Part model, mm, in its own coordinate system. Coordinates: 2 decimals unless noted, no trailing zeros. Order: outer loops, then holes, each group sorted by start corner. A loop starts at its lowest first (then second) coordinate and runs counter-clockwise, first axis right, second up. Notation, with made-up numbers: M 3,-27 L 29,-27 A30 ccw 29,0 Z; hole C 9,-17.75 d11. An arc over 180 degrees is marked long. Answer in a Markdown table with one row per item. Add a question column.
from build123d import *

# Parameters (mm, degrees)
SKETCH1_W               = 279.4
SKETCH1_H               = 76.2
BOSS_EXTRUDE1_DEPTH     = 3
SKETCH3_W               = 3
SKETCH3_H               = 7.8
CUT_EXTRUDE1_DEPTH      = 145.833352512
LPATTERN1_COUNT         = 4
LPATTERN1_PITCH         = 22.8
MIRROR1_COPY_1_SKETCH_W = 3
MIRROR1_COPY_1_SKETCH_H = 7.8
MIRROR1_COPY_1_DEPTH    = 145.833352512
MIRROR1_COPY_2_SKETCH_W = 3
MIRROR1_COPY_2_SKETCH_H = 7.8
MIRROR1_COPY_2_DEPTH    = 145.833352512
MIRROR1_COPY_3_SKETCH_W = 3
MIRROR1_COPY_3_SKETCH_H = 7.8
MIRROR1_COPY_3_DEPTH    = 145.833352512
SKETCH5_W               = 3
SKETCH5_H               = 15
CUT_EXTRUDE3_DEPTH      = 10
SKETCH9_W               = 3
SKETCH9_H               = 7.8
BOSS_EXTRUDE2_DEPTH     = 3
LPATTERN4_COUNT         = 12
LPATTERN4_PITCH         = 22.8


with BuildPart() as part:
    # Sketch1 → Boss-Extrude1 (new body)
    with BuildSketch(Plane(origin=(0, 0, 0), x_dir=(0, 0, -1), z_dir=(1, 0, 0))):
        Rectangle(SKETCH1_W, SKETCH1_H)
    extrude(amount=-BOSS_EXTRUDE1_DEPTH)

    # Sketch3 → Cut-Extrude1 (cut, through all)
    with BuildSketch(Plane.ZY.offset(3)):
        with Locations((-138.2, 34.2)):
            Rectangle(SKETCH3_W, SKETCH3_H)
    cut_extrude1 = extrude(amount=-CUT_EXTRUDE1_DEPTH, mode=Mode.SUBTRACT)

    # LPattern1: Cut-Extrude1 ×4
    with Locations(*[(0, -i * LPATTERN1_PITCH, 0) for i in range(1, LPATTERN1_COUNT)]):
        add(cut_extrude1, mode=Mode.SUBTRACT)

    # Mirror1: Cut-Extrude1 across plane
    add(cut_extrude1.mirror(Plane.XY), mode=Mode.SUBTRACT)

    # Mirror1 copy 1 sketch → Mirror1 copy 1 (cut, through all)
    with BuildSketch(Plane(origin=(-3, -22.8, 0), x_dir=(0, 0, -1), z_dir=(-1, 0, 0))):
        with Locations((-138.2, -34.2)):
            Rectangle(MIRROR1_COPY_1_SKETCH_W, MIRROR1_COPY_1_SKETCH_H)
    extrude(amount=-MIRROR1_COPY_1_DEPTH, mode=Mode.SUBTRACT)

    # Mirror1 copy 2 sketch → Mirror1 copy 2 (cut, through all)
    with BuildSketch(Plane(origin=(-3, -45.6, 0), x_dir=(0, 0, -1), z_dir=(-1, 0, 0))):
        with Locations((-138.2, -34.2)):
            Rectangle(MIRROR1_COPY_2_SKETCH_W, MIRROR1_COPY_2_SKETCH_H)
    extrude(amount=-MIRROR1_COPY_2_DEPTH, mode=Mode.SUBTRACT)

    # Mirror1 copy 3 sketch → Mirror1 copy 3 (cut, through all)
    with BuildSketch(Plane(origin=(-3, -68.4, 0), x_dir=(0, 0, -1), z_dir=(-1, 0, 0))):
        with Locations((-138.2, -34.2)):
            Rectangle(MIRROR1_COPY_3_SKETCH_W, MIRROR1_COPY_3_SKETCH_H)
    extrude(amount=-MIRROR1_COPY_3_DEPTH, mode=Mode.SUBTRACT)

    # Sketch5 → Cut-Extrude3 (cut)
    with BuildSketch(Plane.ZY.offset(3)):
        with Locations((-21.5, 22.8)):
            Rectangle(SKETCH5_W, SKETCH5_H)
    cut_extrude3 = extrude(amount=-CUT_EXTRUDE3_DEPTH, mode=Mode.SUBTRACT)

    # Mirror2: Cut-Extrude3 across plane
    add(cut_extrude3.mirror(Plane.XY), mode=Mode.SUBTRACT)

    # Sketch9 → Boss-Extrude2 (add)
    with BuildSketch(Plane(origin=(0, 38.1, 0), x_dir=(1, 0, 0), z_dir=(0, 1, 0))):
        with Locations((-1.5, 125.4)):
            Rectangle(SKETCH9_W, SKETCH9_H)
    boss_extrude2 = extrude(amount=BOSS_EXTRUDE2_DEPTH)

    # LPattern4: Boss-Extrude2 ×12
    with Locations(*[(0, 0, i * LPATTERN4_PITCH) for i in range(1, LPATTERN4_COUNT)]):
        add(boss_extrude2)


solid = part.part
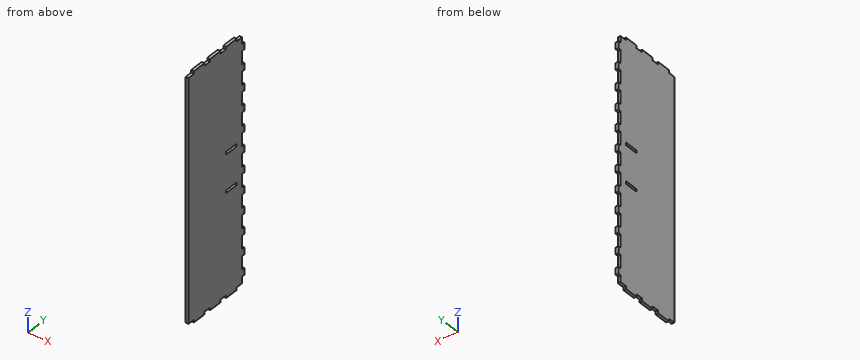
(1) Drop flat-ended pins along their axis: P1, Ø5, axis at y = -2, z = -74.5, coming from the +X side; P2, Ø0.9, axis at x = -2, y = 39.5, coming from the +Z side; P3, Ø1.5, axis at x = -1.5, z = -138.5, coming from the -Y side; P4, Ø0.9, axis at x = -1, z = -21, coming from the +Y side. Give the stop position or say it passes through.
(2) Slice it at A-A (x = -0.6). State how many separate pieces and enclosed holes the cut face has, and give its area (3 significant figures).
(3) Wall check: line 1 (Z direction, x = -2.8, y = 20); line 2 (Y direction, x = -2.1, z = 21.5); line 3 (Z direction, x = -0.5, y = 10). Give the ranges that are in metal, low to high.
(4) Slice it at C-C (y = -10.5). List the corners of the cut face in (x, z), and give its area (3 significant figures).
(5) Slice it at B-B (z = 47). List the corners of the cut face in (x, y).
Computed:
| question | item | result |
|---|---|---|
| 1 | P1 | stops at x = 0 |
| 1 | P2 | stops at z = 129.3 |
| 1 | P3 | stops at y = -30.3 |
| 1 | P4 | stops at y = 38.1 |
| 2 | separate pieces | 1 |
| 2 | enclosed holes | 2 |
| 2 | area | 21,300 mm^2 |
| 3 | line 1 | z = -139.7 to -23, -20 to 20, 23 to 139.7 |
| 3 | line 2 | y = -38.1 to 15.3, 30.3 to 38.1 |
| 3 | line 3 | z = -136.7 to 136.7 |
| 4 | outline | M -3,-136.7 L 0,-136.7 L 0,136.7 L -3,136.7 Z |
| 4 | area | 820 mm^2 |
| 5 | outline | M -3,-38.1 L 0,-38.1 L 0,38.1 L -3,38.1 Z |
